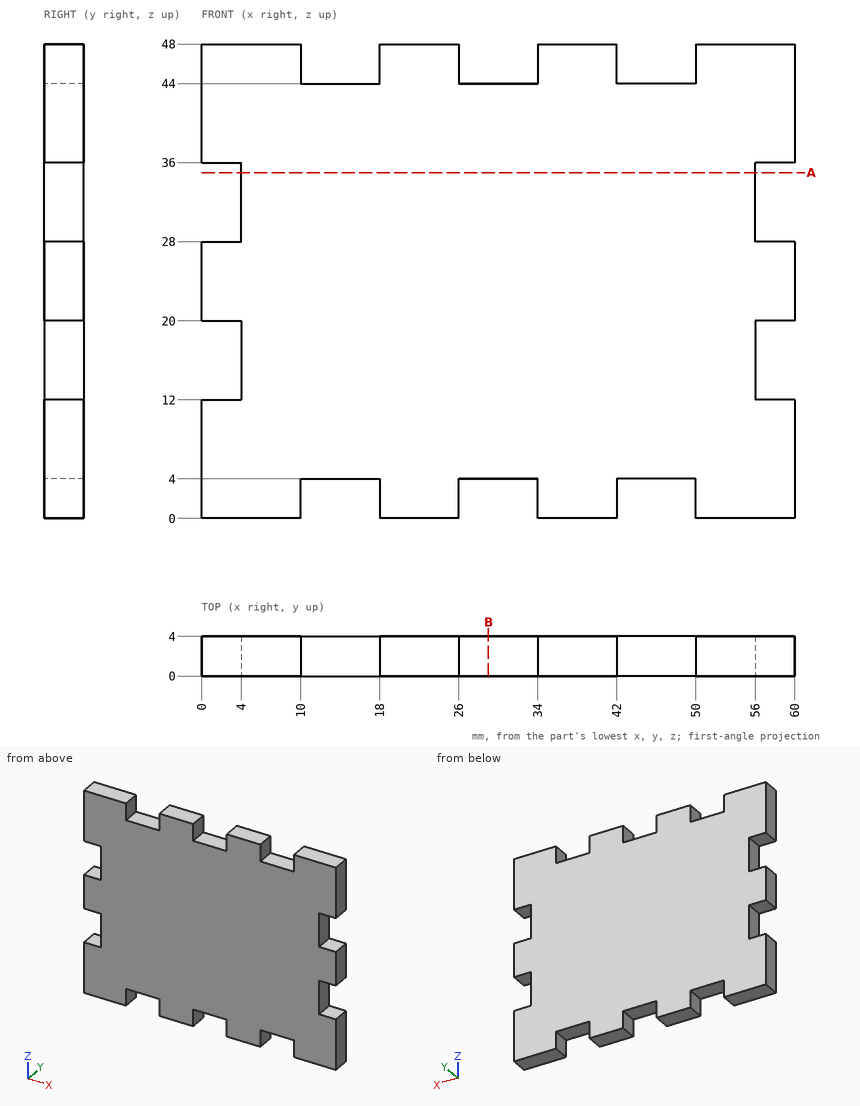
Geometry check sheet. Reference: drawing and pictorial views, mm from the part's lowest x, y, z. Give positions to 0.01 mm unless a question says otherwise; leave off trailing zeros. Order: outer loops, then holes, each group sorted by start corner. A loop starts at its lowest first (then second) coordinate and runs counter-clockwise, first axis right, second up. Notation, with made-up numbers: (76, 16) -> (129, 16) arc R16 ccw to (129, 28) -> close; hole circle Ø5 at (58.5, -29). An arc over 180 degrees is marked (long way). Write each question's results on one line, items separated by ' | '. Start each with the question number.
(1) Sectioned sample at B-B (x = 29). Enter the section's corners in (y, z).
(2) Sectioned sample at A-A (z = 35). Enter the section's corners in (x, y), plus the area to 3 significant figures.
(3) Gauge pin test, flat ends, axial feed: P1, Ø1.2, axis at y = 1, z = 33.5, coming from the -X side; P2, Ø2, axis at y = 3, z = 32.5, coming from the +X side; P3, Ø2, axis at x = 15.5, y = 3, coming from the -Z side. Record the tip position at first contact, or that the pin passes through.
(4) Scan lines: line 1 (X direction, y = 0.5, z = 45); line 2 (Z direction, x = 57.5, y = 3.7); line 3 (Z direction, x = 11.5, y = 2.65). Record each from-to range of solid material in increasing order.
Answer below:
1) outline: (0, 4) -> (4, 4) -> (4, 44) -> (0, 44) -> close
2) outline: (4, 0) -> (56, 0) -> (56, 4) -> (4, 4) -> close | area: 208 mm2
3) P1: x = 4 | P2: x = 56 | P3: z = 4
4) line 1: 0 to 10, 18 to 26, 34 to 42, 50 to 60 | line 2: 0 to 12, 20 to 28, 36 to 48 | line 3: 4 to 44
